Design review of the part shown in the three views and the two pictorial views. Dimensions are in mm from the part's minimum x, y and z. A direction names the side the tool comes from. Give positions to 0.01 mm unless a question says otherwise; leave off trailing zeros. Loops run counter-clockwise (first coordinate to the right, second up) from the corner with the lowest first, then second, coordinate; pieces in that order, holes last. Notation, with made-up numbers: (71, 19) -> (102, 19) arc R28 cw to (102, 38) -> close; hole circle Ø2 at (-17.5, 25). An arc over 180 degrees is marked (long way). Answer as CSV lines item,"result". Start each with the question number.
Item 1: Clearance check with flat-ended pins moving along their axes: P1, Ø10, axis at x = 1336.5, z = 946.5, coming from the +Y side; P2, Ø4, axis at x = 927, y = 587.5, coming from the -Z side; P3, Ø8, axis at y = 1179.5, z = 500, coming from the +X side. State where each tip first meets the part, or that it passes through.
Item 2: For L1, parallel to Y at x = 784, z = 775; L2, parallel to Z at x = 700.5, y = 956.5, list the stretches that pass through material, from the lowest coordinate up. Write a range as from..to.
Item 3: Add section D-D on y = 584. State the section outline as (x, z) points.
Item 4: Add section C-C on z = 949. State the section outline as (x, y) points.
Item 5: Add section B-B on x = 946.5. State the section outline as (y, z) points.
Item 6: Machinability: for the marked faces 1, 2 and 3, which of the approach directions +Z, -Z, +X, -X, +Y, -Y give a long, thin tool a straight path to every point of the face, cutting with its end or side? Answer none if there is none.
Item 7: Add section A-A on y = 234.5. State the section outline as (x, z) points, plus the area to 3 significant figures.
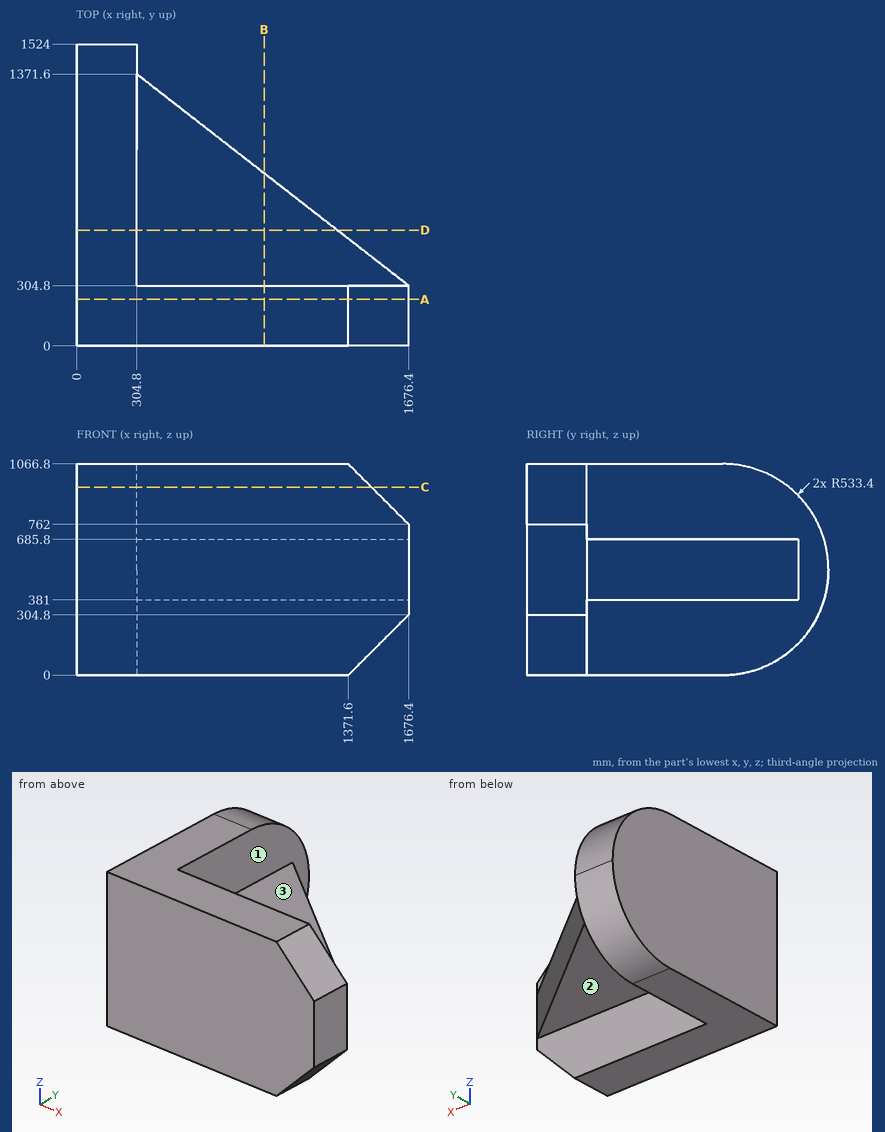
Computed values:
1,P1,"y = 304.8"
1,P2,"z = 381"
1,P3,"x = 556.93"
2,L1,"0..304.8"
2,L2,"381..685.8"
3,outline,"(0, 0) -> (304.8, 0) -> (304.8, 381) -> (1317.43, 381) -> (1317.43, 685.8) -> (304.8, 685.8) -> (304.8, 1066.8) -> (0, 1066.8) -> close"
4,outline,"(0, 0) -> (1489.4, 0) -> (1489.4, 304.8) -> (304.8, 304.8) -> (304.8, 1324.95) -> (0, 1324.95) -> close"
5,outline,"(0, 0) -> (304.8, 0) -> (304.8, 381) -> (872.5, 381) -> (872.5, 685.8) -> (304.8, 685.8) -> (304.8, 1066.8) -> (0, 1066.8) -> close"
6,face 1,"+X, +Y"
6,face 2,"-Z, +X, +Y"
6,face 3,"+Z, +X, +Y"
7,outline,"(0, 0) -> (1371.6, 0) -> (1676.4, 304.8) -> (1676.4, 762) -> (1371.6, 1066.8) -> (0, 1066.8) -> close"
7,area,"1,700,000 mm²"
